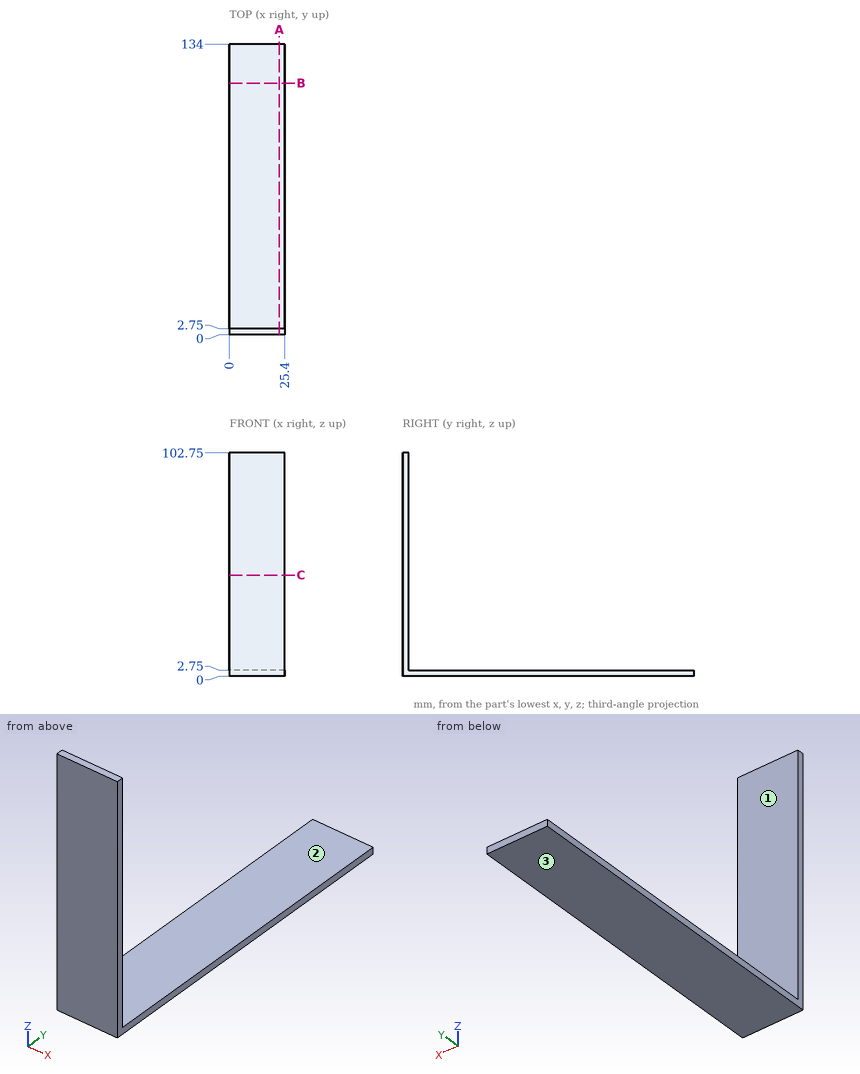
Here's the drawing with two shaded views (mm, measured from the low corner). I have some questions. Give positions to 0.01 mm unless a question says otherwise; leave off trailing zeros. Loops run counter-clockwise (first coordinate to the right, second up) from the corner with the lowest first, then second, coordinate; pieces in that order, holes last. Notation, with made-up numbers: (88, -8.5) -> (115, -8.5) arc R31 cw to (115, 27.5) -> close; hole circle Ø2 at (-38.5, 39). An arc over 180 degrees is marked (long way). Answer as a JSON object with one key per item and string values. Group by question number.
Item 1: Imagine slicing it at A-A on x = 23. Write out the boundary of the cut face in (y, z).
Item 2: Imagine slicing it at B-B on y = 116. Write out the boundary of the cut face in (x, z).
Item 3: I need wall thicknesses on L1, parallel to Y at x = 14, z = 50. Which ranges of the line are inside material? Lowest first, please.
Item 4: Will these pins go through, and if not, where does the flat tip stop? pin 1 (7.5 mm diameter, centred on x = 8.5, z = 56.5, fed in from +Y); pin 2 (12 mm diameter, centred on x = 10.5, y = 80, fed in from -Z); pin 3 (3 mm diameter, centred on x = 11, y = 19.5, fed in from +Z).
Item 5: Thinking about a two-plate mould opening in Z: for the marked faces 1, 2 and 3, which applies, pulls with the +Z half, pulls with the -Z half, needs draft (parallel to the pull), parting line crosses it, or undercut?
Answer list:
{
 "1": {"outline": "(0, 0) -> (134, 0) -> (134, 2.75) -> (2.75, 2.75) -> (2.75, 102.75) -> (0, 102.75) -> close"},
 "2": {"outline": "(0, 0) -> (25.4, 0) -> (25.4, 2.75) -> (0, 2.75) -> close"},
 "3": {"L1": "y = 0 to 2.75"},
 "4": {"pin 1": "stops at y = 2.75", "pin 2": "stops at z = 0", "pin 3": "stops at z = 2.75"},
 "5": {"face 1": "needs draft", "face 2": "pulls with the +Z half", "face 3": "pulls with the -Z half"}
}
